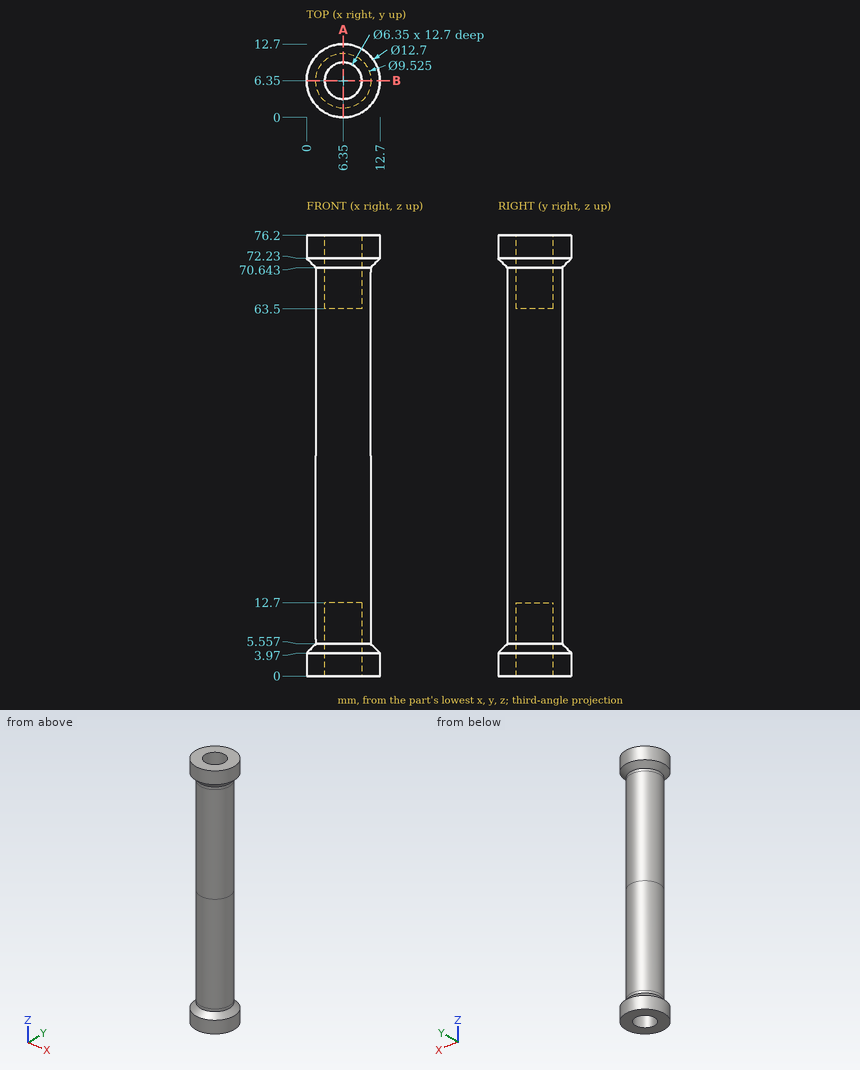
Source: three-view drawing plus pictorial views. Frame: mm from the lowest corner of the part. Give positions to 0.01 mm unless a question says otherwise; leave off trailing zeros. Order: outer loops, then holes, each group sorted by start corner. A loop starts at its lowest first (then second) coordinate and runs counter-clockwise, first axis right, second up.
1. Section A-A on x = 6.35. Return the cut outline in (y, z) (1 decimal), and give its area (3 significant figures).
Derived:
outline: (0, 0) - (3.2, 0) - (3.2, 12.7) - (9.5, 12.7) - (9.5, 0) - (12.7, 0) - (12.7, 4) - (11.1, 5.6) - (11.1, 70.6) - (12.7, 72.2) - (12.7, 76.2) - (9.5, 76.2) - (9.5, 63.5) - (3.2, 63.5) - (3.2, 76.2) - (0, 76.2) - (0, 72.2) - (1.6, 70.6) - (1.6, 5.6) - (0, 4) - close
area: 595 mm2
2. Pin query (flat end, axial travel): pin 1 (5 mm diameter, centred on x = 8, z = 55.5, fed in from -Y); pin 2 (2 mm diameter, centred on x = 8.5, y = 3.5, fed in from -Z); pin 3 (6 mm diameter, centred on y = 2.5, z = 29, fed in from -X); pin 4 (4 mm diameter, centred on x = 8, z = 42, fed in from +Y). Return the tip coordinate at first contact, or that it passes through.
Derived:
pin 1: stops at y = 1.59
pin 2: stops at z = 0
pin 3: stops at x = 1.66
pin 4: stops at y = 11.11
3. Material intervals for L1, parallel to Y at x = 6.35, z = 67 (1 decimal); L2, parallel to Z at x = 5.25, y = 5, sorted ascending.
Derived:
L1: y = 1.6 to 3.2, 9.5 to 11.1
L2: z = 12.7 to 63.5
